Source: three-view drawing plus pictorial views. Frame: mm from the lowest corner of the part. A direction names the side the tool comes from. Give positions to 0.01 mm unless a question says otherwise; leave off trailing zeros. Order: outer loops, then holes, each group sorted by start corner. A loop starts at its lowest first (then second) coordinate and runs counter-clockwise, first axis right, second up. Notation, with made-up numbers: (57.5, -36) - (89.5, -36) arc R19 ccw to (89.5, -12) - close; hole circle Ø1 at (73, 43). An arc over 180 degrees is marked (long way). Use CSV: the item, a comma, the result in double quotes.
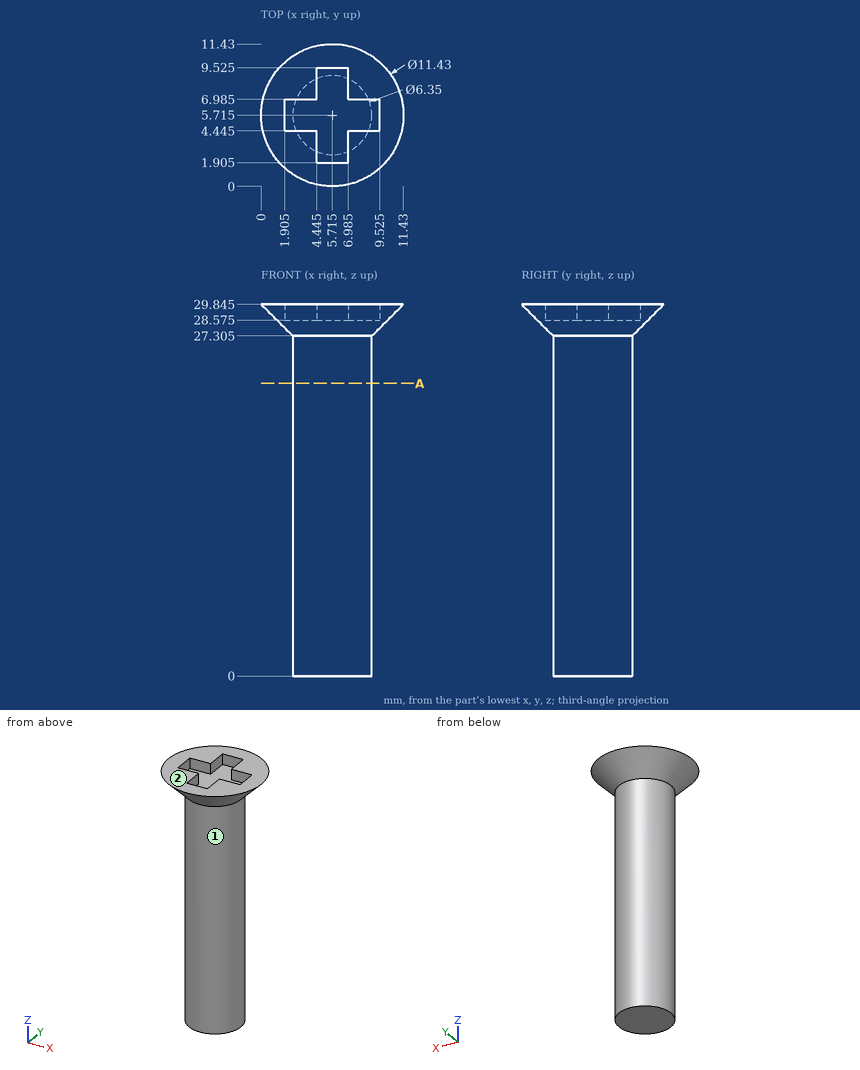
Item 1: First-contact query: pin 1 (1.5 mm diameter, centred on y = 9, z = 9, fed in from -X); pin 2 (0.6 mm diameter, centred on x = 5.5, z = 29, fed in from -Y); pin 3 (1.4 mm diameter, centred on y = 3, z = 29.5, fed in from -X). Flat tips, straight axial feed; report the tip coordinate or a pass-through.
Filled in:
pin 1,"stops at x = 3.8"
pin 2,"stops at y = 0.55"
pin 3,"stops at x = 0.4"
Item 2: Material intervals for line 1 (Z direction, x = 6, y = 4.25) (3 decimals); line 2 (Y direction, x = 8, z = 19); line 3 (X direction, y = 4, z = 2.5), sorted ascending. Write a range as from..to.
Filled in:
line 1,"z = 0..28.575"
line 2,"y = 3.51..7.92"
line 3,"x = 3.04..8.39"
Item 3: Section A-A on z = 23.5. Return the cut outline in (x, y) (3 decimals), then the cut area to 3 significant figures.
Filled in:
outline,"circle Ø6.35 at (5.715, 5.715)"
area,"31.7 mm2"
Item 4: Set-up query: the marked faces 1 and 2. Return all of +Z, -Z, +X, -X, +Y, -Y with unobstructed straight access to the full face (end or side cutting, diameter ignored); none if empty.
Filled in:
face 1,"-Z"
face 2,"+Z, +X, -X, +Y, -Y"
